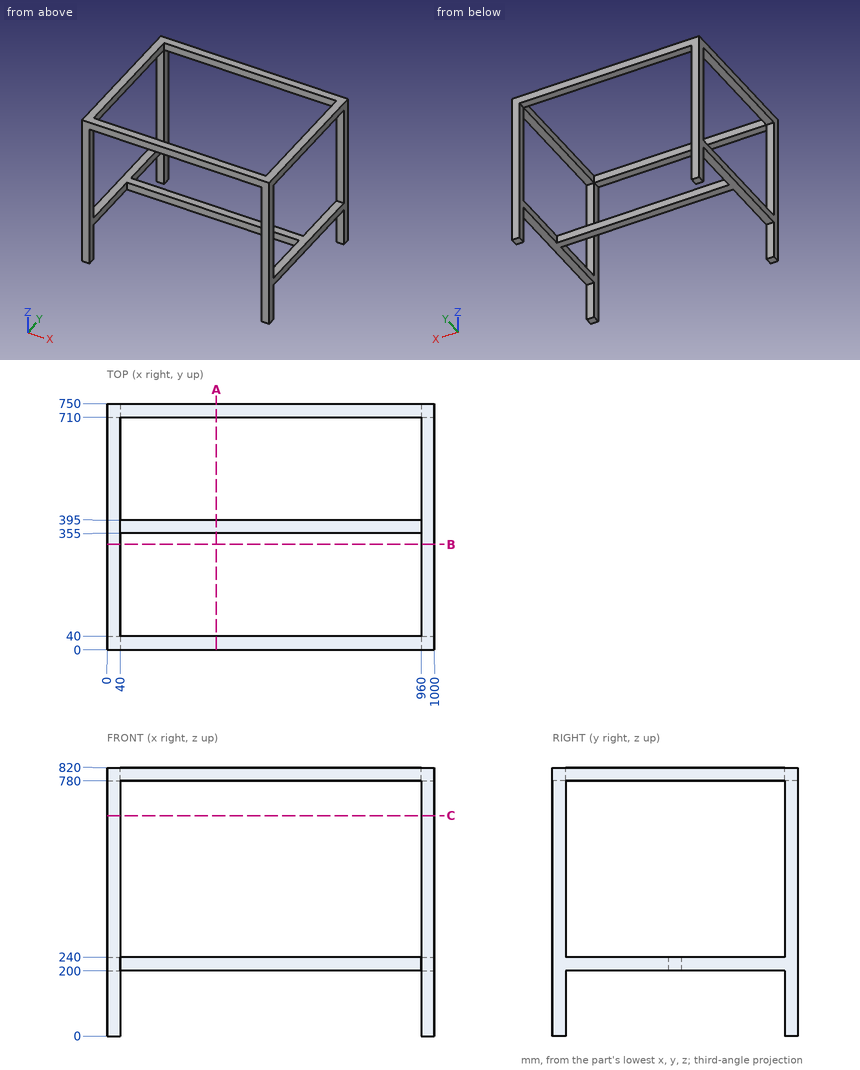
Job drawing, mm, ordinate dimensions from the low corner. One solid piece. Give positions to 0.01 mm unless a question says otherwise; leave off trailing zeros. Order: outer loops, then holes, each group sorted by start corner. A loop starts at its lowest first (then second) coordinate and runs counter-clockwise, first axis right, second up. Notation, with made-up numbers: M -29.75,-23 L -6.75,-23 A26 cw -6.75,-2 Z; hole C 72.25,65 d5. An arc over 180 degrees is marked long. Put each result on its own line as item: value. Start each with the question number.
(1) Band-saw the part on A-A on x = 334. Give the cut face in (y, z), then the cut area to 3 significant figures.
(2) Band-saw the part on B-B on y = 321.5. Give the cut face in (x, z), then the cut area to 3 significant figures.
(3) Band-saw the part on C-C on z = 673.5. Give the cut face in (x, y), then the cut area to 3 significant figures.
(4) Pin check, flat tip, straight feed: pin 1 Ø12 at (x, y) = (12.5, 484.5) entering from -Z. Stop position of the tip, or through.
(5) Drill centre lines: L1, parallel to X at y = 209.5, z = 783; L2, parallel to Z at x = 367.5, y = 384. Where is each one in solid material? Low to high. Write a range as [from, to].
Results below:
1. outline: M 0,780 L 40,780 L 40,820 L 0,820 Z; M 355,200 L 395,200 L 395,240 L 355,240 Z; M 710,780 L 750,780 L 750,820 L 710,820 Z
1. area: 4,800 mm2
2. outline: M 0,200 L 40,200 L 40,240 L 0,240 Z; M 0,780 L 40,780 L 40,820 L 0,820 Z; M 960,200 L 1000,200 L 1000,240 L 960,240 Z; M 960,780 L 1000,780 L 1000,820 L 960,820 Z
2. area: 6,400 mm2
3. outline: M 0,0 L 40,0 L 40,40 L 0,40 Z; M 0,710 L 40,710 L 40,750 L 0,750 Z; M 960,0 L 1000,0 L 1000,40 L 960,40 Z; M 960,710 L 1000,710 L 1000,750 L 960,750 Z
3. area: 6,400 mm2
4. pin 1: stops at z = 200
5. L1: x = [0, 40], [960, 1000]
5. L2: z = [200, 240]
